For this review, take the finished solid that the model builds, in its own axes (mm). A direction names the side the tool comes from. Round coordinates to 2 decimals unless told otherwise and drop trailing zeros. Order: outer loops, then holes, each group sorted by start corner. A loop starts at its lowest first (then second) coordinate and runs counter-clockwise, first axis right, second up. Notation, with made-up numbers: M -39,46 L -25,46 A15 cw -25,71 Z; hole C 8.5,64.5 d5. An arc over 180 degrees is marked long. Answer as a JSON object with one key per item and string values.
from build123d import *

# Parameters (mm, degrees)
SKETCH1_W           = 480
SKETCH1_H           = 250
BOSS_EXTRUDE1_DEPTH = 70
SKETCH2_W           = 250
SKETCH2_H           = 20
BOSS_EXTRUDE2_DEPTH = 50
CHAMFER1_SIZE       = 55
CHAMFER1_SIZE_2     = 51.288329738
SKETCH3_W           = 250
SKETCH3_H           = 20
BOSS_EXTRUDE3_DEPTH = 20
CHAMFER3_SIZE       = 56
CHAMFER3_SIZE_2     = 20.382333119
SHELL1_START        = -115
SHELL1_DEPTH        = 230
SKETCH4_R           = 3
BOSS_EXTRUDE4_DEPTH = 5
SKETCH6_R           = 3
BOSS_EXTRUDE5_DEPTH = 10


# Read off the part's stored shape, not the designer's step: Shell1
with BuildPart() as part:
    # Sketch1 → Boss-Extrude1 (new body)
    with BuildSketch(Plane(origin=(0, 0, 0), x_dir=(1, 0, 0), z_dir=(0, 1, 0))):
        Rectangle(SKETCH1_W, SKETCH1_H)
    extrude(amount=BOSS_EXTRUDE1_DEPTH)

    # Sketch2 → Boss-Extrude2 (add)
    with BuildSketch(Plane.ZY.offset(240)):
        with Locations((0, 60)):
            Rectangle(SKETCH2_W, SKETCH2_H)
    extrude(amount=BOSS_EXTRUDE2_DEPTH)

    # Chamfer1
    # the kernel refuses this chamfer: 55, 51.288329738 mm, written as the material it adds along each edge
    with BuildSketch(Plane(origin=(-240, 50, 125), x_dir=(0.02649526118620358, -0.9996489389454054, 0), z_dir=(0, 0, -1))) as chamfer1_piece_1_section:
        Polygon((CHAMFER1_SIZE * 0.999648938945, CHAMFER1_SIZE * 0.0264952611862), (-CHAMFER1_SIZE_2 * 0.026495261186, CHAMFER1_SIZE_2 * 0.999648938937), (0, 0), align=None)
    chamfer1_piece_1 = extrude(amount=250, mode=Mode.PRIVATE)
    chamfer1_piece_1 = split(chamfer1_piece_1, bisect_by=Plane(origin=(-257.002695591, 0, 0), z_dir=(0, 1, 0)), keep=Keep.TOP, mode=Mode.PRIVATE)
    chamfer1_piece_1 = split(chamfer1_piece_1, bisect_by=Plane(origin=(-290, 32.326466584, 0), z_dir=(1, 0, 0)), keep=Keep.TOP, mode=Mode.PRIVATE)
    add(chamfer1_piece_1)

    # Sketch3 → Boss-Extrude3 (add)
    with BuildSketch(Plane(origin=(240, 0, 0), x_dir=(0, 0, -1), z_dir=(1, 0, 0))):
        with Locations((0, 60)):
            Rectangle(SKETCH3_W, SKETCH3_H)
    extrude(amount=BOSS_EXTRUDE3_DEPTH)

    # Chamfer3
    # the kernel refuses this chamfer: 56, 20.382333119 mm, written as the material it adds along each edge
    with BuildSketch(Plane(origin=(240, 50, -125), x_dir=(-0.013184058198645885, -0.9999130865277316, 0), z_dir=(0, 0, 1))) as chamfer3_piece_1_section:
        Polygon((CHAMFER3_SIZE * 0.999913086528, CHAMFER3_SIZE * 0.0131840581986), (-CHAMFER3_SIZE_2 * 0.0131840581986, CHAMFER3_SIZE_2 * 0.999913086523), (0, 0), align=None)
    chamfer3_piece_1 = extrude(amount=250, mode=Mode.PRIVATE)
    chamfer3_piece_1 = split(chamfer3_piece_1, bisect_by=Plane(origin=(246.40635993, 0, 0), z_dir=(0, 1, 0)), keep=Keep.TOP, mode=Mode.PRIVATE)
    chamfer3_piece_1 = split(chamfer3_piece_1, bisect_by=Plane(origin=(260, 31.786057297, 0), z_dir=(-1, 0, 0)), keep=Keep.TOP, mode=Mode.PRIVATE)
    add(chamfer3_piece_1)

    # Shell1 outline → Shell1 (cut)
    with BuildSketch(Plane.XY.offset(SHELL1_START)):
        Polygon((-242.488513556, 5), (238.682783715, 5), (250, 36.093796195), (250, 70), (-280, 70), (-280, 45.226144329), align=None)
    extrude(amount=SHELL1_DEPTH, mode=Mode.SUBTRACT)

    # Sketch4 → Boss-Extrude4 (add)
    with BuildSketch(Plane.XY.offset(125)):
        with Locations(Location((220, 60, 0), (0, 0, 180))):
            Circle(SKETCH4_R)
        with Locations(Location((140, 60, 0), (0, 0, 180))):
            Circle(SKETCH4_R)
        with Locations(Location((60, 60, 0), (0, 0, 180))):
            Circle(SKETCH4_R)
        with Locations(Location((-20, 60, 0), (0, 0, 180))):
            Circle(SKETCH4_R)
        with Locations(Location((-100, 60, 0), (0, 0, 180))):
            Circle(SKETCH4_R)
        with Locations(Location((-180, 60, 0), (0, 0, 180))):
            Circle(SKETCH4_R)
    extrude(amount=BOSS_EXTRUDE4_DEPTH)

    # Sketch6 → Boss-Extrude5 (add)
    with BuildSketch(Plane.XY.offset(125)):
        with Locations(Location((160, 10, 0), (0, 0, 180))):
            Circle(SKETCH6_R)
        with Locations(Location((80, 10, 0), (0, 0, 180))):
            Circle(SKETCH6_R)
        with Locations(Location((0, 10, 0), (0, 0, 180))):
            Circle(SKETCH6_R)
        with Locations(Location((-80, 10, 0), (0, 0, 180))):
            Circle(SKETCH6_R)
        with Locations(Location((-160, 10, 0), (0, 0, 180))):
            Circle(SKETCH6_R)
        with Locations(Location((-240, 10, 0), (0, 0, 180))):
            Circle(SKETCH6_R)
    extrude(amount=BOSS_EXTRUDE5_DEPTH)


solid = part.part
1) For L1, parallel to Z at x = -19, y = 38; L2, parallel to X at y = 60, z = -23; L3, parallel to Y at x = 21, z = 84.5, list the stretches that pass through material, from the lowest coordinate up.
Geometry check:
{"L1": "z = -125 to -115, 115 to 125", "L2": "x = -290 to -280, 250 to 260", "L3": "y = 0 to 5"}
2) Insertion check: P1, Ø19.5, axis at x = 75, y = 22, coming from the +Z side; P2, Ø12, axis at x = -191, z = 60.5, coming from the +Y side; P3, Ø3, axis at x = -20.5, y = 58.5, coming from the +Z side. Each pin has a flat end and moves straight along its axis. Give the tip position at first contact, or say it passes through.
Geometry check:
{"P1": "stops at z = 125", "P2": "stops at y = 5", "P3": "stops at z = 130"}
3) Mouldability with a two-part tool opening along X and no side actions: class faces 3 (the flat face through (-280, 58, -2)), 4 (the flat face through (-98, 70, 121)), 5 (the flat face through (250, 53, -2)), 6 (the flat face through (-267.014, 23.969, 1.75)) as +X half, -X half, draft (parallel to the pull), parting line (faces both ways), or undercut.
Geometry check:
{"face 3": "undercut", "face 4": "draft", "face 5": "undercut", "face 6": "-X half"}
4) Add section B-B on x = -190. State the section outline as (y, z) points.
Geometry check:
{"outline": "M 0,-125 L 70,-125 L 70,-115 L 5,-115 L 5,115 L 70,115 L 70,125 L 0,125 Z"}
5) Machinability: for faces 1 (the flat face through (2, 0, -2)), 2 (the flat face through (-19, 38, -115)), which of the approach directions +Z, -Z, +X, -X, +Y, -Y give a long, thin tool a straight path to every point of the face, cutting with its end or side? Answer none if there is none.
Geometry check:
{"face 1": "+Z, -Z, +X, -X, -Y", "face 2": "+Y"}
6) Add section A-A on z = 29.5. State the section outline as (x, y) points, and give its area (3 significant figures).
Geometry check:
{"outline": "M -290,48.62 L -244.66,0 L 242.18,0 L 260,48.95 L 260,70 L 250,70 L 250,36.09 L 238.68,5 L -242.49,5 L -280,45.23 L -280,70 L -290,70 Z", "area": "3,440 mm²"}
